from build123d import *

# Parameters (mm, degrees)
F1_DEPTH    = 508
F3_DEPTH    = 177.8
F4_T        = 3.175
F4_T3_DEPTH = 111.0768828907
F4_T5_DEPTH = 57.15
F4_T7_DEPTH = 111.0768828907
F6_DEPTH    = 25.4
F8_DEPTH    = 25.4


# Not quite as in the source:
# - a shell that OpenCascade refuses in one call is made with other operations: the cavity is built on its own and cut out


with BuildPart() as f1:
    # F0 (on Front) → F1 (new body)
    with BuildSketch(Plane.XZ):
        Polygon((-25.4, 0), (0, 0), (25.4, 0), (50.8, 101.6), (-50.8, 101.6), align=None)
    extrude(amount=-F1_DEPTH)

    # F2 (on Front) → F3 (join)
    with BuildSketch(Plane.XZ):
        Polygon((76.2, -101.6), (76.2, 0), (76.2, 101.6), (-76.2, 101.6), (-76.2, 0), (-76.2, -101.6), align=None)
    extrude(amount=F3_DEPTH)

    # F4: shell of thickness 3.175, made by hand


with BuildPart() as f4_core1:
    # F4_t2: copy of F1
    add(f1.part)

    # the walls: a layer under each face that stays
    f4_faces = [f4_core1.faces().sort_by_distance(p)[0] for p in [
        (76.2, -88.9, 0),
        (0, -88.9, -101.6),
        (0, -177.8, 0),
        (-50.8, 0, -67.7333333333),
        (-76.2, -88.9, 0),
        (-38.1, 254, 50.8),
        (0, 254, 0),
        (38.1, 254, 50.8),
        (0, 508, 50.8),
    ]]
    thicken(f4_faces, amount=-F4_T, mode=Mode.SUBTRACT)

    # F4_s4 → F4_t3 (cut)
    with BuildSketch(Plane(origin=(-27.6641682565, 0, 110.6566730262), x_dir=(0, 1, 0), z_dir=(0.242535625, 0, -0.9701425001))):
        Polygon((0.03175, -24.6733695037), (-3.175, -24.6416195037), (-3.175, -21.4666195037), (0, -21.4666195037), align=None)
    extrude(amount=F4_T3_DEPTH, mode=Mode.SUBTRACT)

    # F4_s6 → F4_t5 (cut)
    with BuildSketch(Plane.YZ.offset(-28.575)):
        Polygon((0.03175, -0.03175), (-3.175, 0), (-3.175, 3.175), (0, 3.175), align=None)
    extrude(amount=F4_T5_DEPTH, mode=Mode.SUBTRACT)

    # F4_s8 → F4_t7 (cut)
    with BuildSketch(Plane(origin=(0.7240670376, 0, 2.8962681503), x_dir=(0, 1, 0), z_dir=(0.242535625, 0, 0.9701425001))):
        Polygon((0.03175, -24.6733695037), (-3.175, -24.6416195037), (-3.175, -21.4666195037), (0, -21.4666195037), align=None)
    extrude(amount=F4_T7_DEPTH, mode=Mode.SUBTRACT)


with BuildPart() as f1_1:
    add(f1.part)

    # what is left inside the walls is the cavity
    f4_cavity = [f4_core1.part.solids().sort_by_distance(p)[0] for p in [
        (0, 51.858333, 101.56825),
    ]]
    add(f4_cavity, mode=Mode.SUBTRACT)

    # F5 (on face) → F6 (cut)
    with BuildSketch(Plane(origin=(0, 508, 0), x_dir=(-1, 0, 0), z_dir=(0, 1, 0))):
        Polygon((-47.5272849097, 101.6), (-50.8, 101.6), (-50.00625, 98.425), (-25.4, 0), (25.4, 0), (50.00625, 98.425), (50.8, 101.6), (47.5272849097, 101.6), (46.7335349097, 98.425), (22.9210349097, 3.175), (-22.9210349097, 3.175), (-46.7335349097, 98.425), align=None)
        Polygon((47.5272849097, 101.6), (-47.5272849097, 101.6), (-46.7335349097, 98.425), (-22.9210349097, 3.175), (22.9210349097, 3.175), (46.7335349097, 98.425), align=None)
    extrude(amount=-F6_DEPTH, mode=Mode.SUBTRACT)

    # F7 (on face) → F8 (cut)
    with BuildSketch(Plane.XZ.offset(177.8)):
        Polygon((-38.1, -12.7), (0, -12.7), (38.1, -12.7), (38.1, 101.6), (-38.1, 101.6), align=None)
    extrude(amount=-F8_DEPTH, mode=Mode.SUBTRACT)


solid = f1_1.part
Model file for the job. Use its own axes, mm. A direction names the side the tool comes from. Coordinates: 2 decimals unless noted, no trailing zeros. Loops run counter-clockwise (first coordinate to the right, second up) from the corner with the lowest first, then second, coordinate; pieces in that order, holes last. Notation, with made-up numbers: (60, 12) -> (79, 12) arc R23 cw to (79, 44) -> close; hole circle Ø2 at (40.25, -17). An arc over 180 degrees is marked (long way). Use one line per item in the form item = value. Start each with the question number.
(1) Cut at B-B on z = 85.5. Give the cut face in (x, y) (3 decimals).
(2) Tool access for faces 4 (the flat face through (73.025, -88, 0)), 5 (the flat face through (-38.278, 237.922, 51.511)), 6 (the flat face through (-1, 0, -21)), 7 (the flat face through (0, 236, 3.175)), 8 (the flat face through (37.922, 237.922, 50.089)): list every direction of +Z, -Z, +X, -X, +Y, -Y with a clear straight run to the whole face (end or side of a thin tool).
(3) Cut at C-C on x = 66. Give the cut face in (y, z) (3 decimals), and give its area (3 significant figures).
(4) Flat gauge pins, fed straight in: pin 1 (14 mm diameter, centred on x = -5.5, y = 342, fed in from +Z) (3 decimals); pin 2 (8 mm diameter, centred on y = 249.5, z = 41.5, fed in from -X) (3 decimals); pin 3 (3 mm diameter, centred on y = 225, z = 56.5, fed in from -X); pin 4 (10 mm diameter, centred on x = 18.5, z = 15.5, fed in from -Y). Where does each tip first touch, or does it go through?
(5) Cut at A-A on z = -81.5. Give the cut face in (x, y) (3 decimals), and give its area (3 significant figures).
(6) Cut at D-D on y = -102. Give the cut face in (x, z) (3 decimals), and give its area (3 significant figures).
(7) Probe probe 1 along X at (y, z) = (-70, 75) (3 decimals); probe 2 along Y at (x, z) = (-18.5, -89.5) (3 decimals); probe 3 along Z at (x, y) = (-38, -54) (3 decimals). List the from-to ranges inside material, lowest first. Write a range as from..to.
(8) Pull direction Y, two halves, no side cores. Call faces 1 (the flat face through (0, 238, 0)), 2 (the flat face through (-1, -3.175, -19)), 3 (the flat face through (30.34, 482.6, 32.22)): pulls with the +Y half, pulls with the -Y half, needs draft (parallel to the pull), parting line crosses it, or undercut.
Values:
q1.outline = (-76.2, -177.8) -> (-38.1, -177.8) -> (-38.1, -174.625) -> (-73.025, -174.625) -> (-73.025, -3.175) -> (-43.502, -3.175) -> (-43.502, 482.6) -> (-46.775, 482.6) -> (-46.775, 0) -> (-76.2, 0) -> close; (38.1, -177.8) -> (76.2, -177.8) -> (76.2, 0) -> (46.775, 0) -> (46.775, 482.6) -> (43.502, 482.6) -> (43.502, -3.175) -> (73.025, -3.175) -> (73.025, -174.625) -> (38.1, -174.625) -> close
q2.face_4 = +Z
q2.face_5 = -Z, -X, +Y
q2.face_6 = -Z, +Y
q2.face_7 = +Z, +Y, -Y
q2.face_8 = -Z, +X, +Y
q3.outline = (-177.8, -101.6) -> (0, -101.6) -> (0, 101.6) -> (-3.175, 101.6) -> (-3.175, -98.425) -> (-174.625, -98.425) -> (-174.625, 101.6) -> (-177.8, 101.6) -> close
q3.area = 1,830 mm2
q4.pin_1 = 3.175
q4.pin_2 = -36.775
q4.pin_3 = -39.9
q4.pin_4 = through
q5.outline = (-76.2, -177.8) -> (76.2, -177.8) -> (76.2, 0) -> (-76.2, 0) -> close; hole (-73.025, -174.625) -> (73.025, -174.625) -> (73.025, -3.175) -> (-73.025, -3.175) -> close
q5.area = 2,060 mm2
q6.outline = (-76.2, -101.6) -> (76.2, -101.6) -> (76.2, 101.6) -> (73.025, 101.6) -> (73.025, -98.425) -> (-73.025, -98.425) -> (-73.025, 101.6) -> (-76.2, 101.6) -> close
q6.area = 1,750 mm2
q7.probe_1 = -76.2..-73.025, 73.025..76.2
q7.probe_2 = -177.8..-174.625, -3.175..0
q7.probe_3 = -101.6..-98.425
q8.face_1 = needs draft
q8.face_2 = undercut
q8.face_3 = pulls with the +Y half
